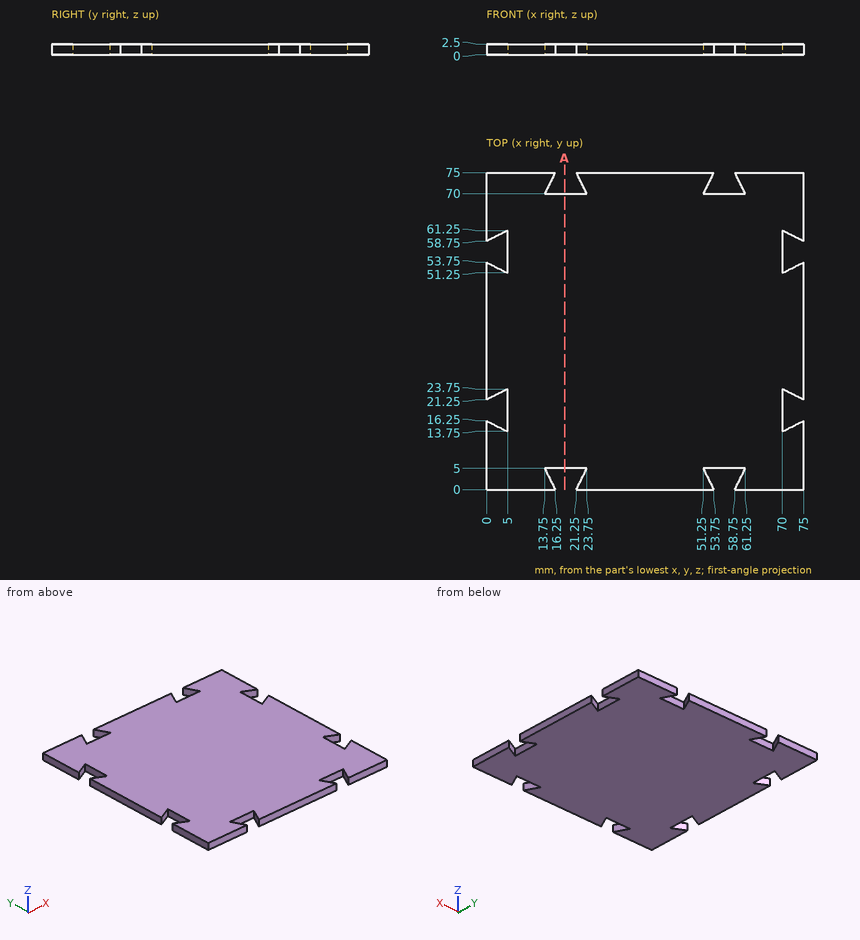
Source: three-view drawing plus pictorial views. Frame: mm from the lowest corner of the part. Give positions to 0.01 mm unless a question says otherwise; leave off trailing zeros. Write each loop counter-clockwise with the first axis right and the second up, starting at its lowest first coordinate (ties: lowest second). Pieces come first, ordered by that corner, then holes.
(1) First-contact query: P1, Ø2, axis at x = 20, y = 66, coming from the -Z side; P2, Ø1.2, axis at x = 58, z = 1, coming from the +Y side; P3, Ø0.8, axis at x = 19.5, z = 2, coming from the -Y side. Flat tips, straight axial feed; report the tip coordinate or a pass-through.
(2) Cut plane A-A, the plane x = 18.5. Return loops of the section in (y, z).
(3) Ray query, line 1 (X direction, y = 15.5, z = 0.6); line 2 (Y direction, x = 16.5, z = 1.75). Return the intervals inside material, ascending.
Values follow:
1. P1: stops at z = 0
1. P2: stops at y = 70
1. P3: stops at y = 5
2. outline: (5, 0) - (70, 0) - (70, 2.5) - (5, 2.5) - close
3. line 1: x = 0 to 1.5, 5 to 70, 73.5 to 75
3. line 2: y = 5 to 70
